Build history of the part. All positions in model axes, mm. A direction names the side the tool comes from. Round coordinates to 2 decimals unless told otherwise and drop trailing zeros. Loops run counter-clockwise (first coordinate to the right, second up) from the corner with the lowest first, then second, coordinate; pieces in that order, holes last. Notation, with made-up numbers: M -21.5,59 L 3.5,59 A27 ccw 3.5,81 Z; hole C 87.25,-20.5 d11. An arc over 180 degrees is marked long. One line per item, written item: value.
```python
from build123d import *

# Parameters (mm, degrees)
F0_W     = 112.955294
F0_H     = 111.52909
F1_DEPTH = 93.472
F2_W     = 112.955294
F2_H     = 111.52909
F3_DEPTH = 13.462
F4_R     = 51.751528
F5_DEPTH = 131.318
F6_R     = 52.996706
F7_DEPTH = 25.4


with BuildPart() as f1:
    # F0 (on Top) → F1 (new body)
    with BuildSketch(Plane.XY):
        with Locations((1.426205, 0.285242)):
            Rectangle(F0_W, F0_H)
    extrude(amount=F1_DEPTH)

    # F2 (on face) → F3 (join)
    with BuildSketch(Plane.XY.offset(93.472)):
        with Locations((1.426205, 0.285242)):
            Rectangle(F2_W, F2_H)
    extrude(amount=F3_DEPTH)

    # F4 (on face) → F5 (cut)
    with BuildSketch(Plane.XY.offset(106.934)):
        Circle(F4_R)
    extrude(amount=-F5_DEPTH, mode=Mode.SUBTRACT)

    # F6 (on face) → F7 (cut)
    with BuildSketch(Plane.XZ.offset(55.479303)):
        with Locations((0, 53.242445)):
            Circle(F6_R)
    extrude(amount=-F7_DEPTH, mode=Mode.SUBTRACT)


solid = f1.part
```
Item 1: Wall check: line 1 along X through (y, z) = (45.5, 64); line 2 along X through (y, z) = (-21, 101); line 3 along Y through (x, z) = (46.5, 46). Give the ranges that are in metal, low to high.
Check values:
line 1: x = -55.05 to -24.66, 24.66 to 57.9
line 2: x = -55.05 to -47.3, 47.3 to 57.9
line 3: y = -30.08 to -22.71, 22.71 to 56.05
Item 2: Slice it at A-A, the plane y = 0. Give the cut face in (x, z).
Check values:
outline: M -55.05,0 L -51.75,0 L -51.75,106.93 L -55.05,106.93 Z; M 51.75,0 L 57.9,0 L 57.9,106.93 L 51.75,106.93 Z
Item 3: Drop flat-ended pins along their axis: P1, Ø3.5, axis at x = -45, z = 57.5, coming from the -Y side; P2, Ø2, axis at x = -6, z = 80.5, coming from the -Y side. Give the stop position or say it passes through.
Check values:
P1: stops at y = -30.08
P2: stops at y = 51.28
Item 4: Slice it at B-B, the plane x = 0. Give the cut face in (y, z), and give its area (3 significant figures).
Check values:
outline: M -55.48,0 L -51.75,0 L -51.75,0.25 L -55.48,0.25 Z; M -55.48,106.24 L -51.75,106.24 L -51.75,106.93 L -55.48,106.93 Z; M 51.75,0 L 56.05,0 L 56.05,106.93 L 51.75,106.93 Z
area: 463 mm2
Item 5: Which spindle directions (+Z, -Z, +X, -X, +Y, -Y) get a long thin tool onto all of the face, cutting with end or side? Do faces 1 (the face through (1, 56.05, 53)), 2 (the face through (46, -30.079, 54)). Say none if no direction does.
Check values:
face 1: +Z, -Z, +X, -X, +Y
face 2: -Y
Item 6: Slice it at C-C, the plane x = -44. Give the cut face in (y, z).
Check values:
outline: M -55.48,0 L -27.24,0 L -27.24,106.93 L -55.48,106.93 L -55.48,82.78 L -30.08,82.78 L -30.08,23.7 L -55.48,23.7 Z; M 27.24,0 L 56.05,0 L 56.05,106.93 L 27.24,106.93 Z
Item 7: Slice it at D-D, the plane z = 97.5. Give the cut face in (x, y), and give its area (3 significant figures).
Check values:
outline: M -55.05,-55.48 L -29.15,-55.48 L -29.15,-42.76 A51.75 cw long 29.15,-42.76 L 29.15,-55.48 L 57.9,-55.48 L 57.9,56.05 L -55.05,56.05 Z
area: 3,800 mm2
Item 8: Pull direction Y, two halves, no side cores. Call faces 3 (the face through (51, -55.479, 69)), 4 (the face through (-6.74, 51.31, 54.22)), 5 (the face through (43, 29.5, 106.934)): pulls with the +Y half, pulls with the -Y half, needs draft (parallel to the pull), parting line crosses it, or undercut.
Check values:
face 3: pulls with the -Y half
face 4: undercut
face 5: needs draft
